Study the drawing (mm; zero at the part's minimum x, y, z) and answer. A direction names the side the tool comes from. Coordinates: 2 decimals unless noted, no trailing zeros. Order: outer loops, then holes, each group sorted by start corner. A loop starts at its lowest first (then second) coordinate and runs counter-clockwise, first axis right, second up.
1. The part is cut by section C-C, the plane y = 2.5. Give the vertices of the cut face in (x, z).
2. The part is cut by section A-A, the plane z = 4.25. Give the vertices of the cut face in (x, y).
3. The part is cut by section D-D, the plane x = 41.5. Give the vertices of the cut face in (y, z), then the cut area to 3 significant figures.
4. The part is cut by section B-B, the plane y = 17.2. Give the vertices of the cut face in (x, z).
5. Find the intervals of material crossed by probe 1 along Z at (x, y) = (2.65, 17.2); probe 2 along X at (y, z) = (9.75, 1.5); probe 3 along Z at (x, y) = (10, 3.5), in increasing order.
6. Determine the mould class of the marked faces 3, 4 and 5 for opening direction X: +X half, -X half, draft (parallel to the pull), parting line (faces both ways), or undercut.
7. A tool of negligible diameter and unlimited length cuts with its end or side. For the marked faces 1 and 2, from which of +Z, -Z, +X, -X, +Y, -Y can it reach the whole face along a straight path? Write none if from no direction.
8. Flat-ended cylindrical pins translate along their axes: pin 1 Ø5 at (x, z) = (42, 4.5) entering from +Y; pin 2 Ø3 at (x, y) = (35, 2.5) entering from -Z; pin 3 Ø4 at (x, z) = (32.5, 5) entering from +Y; pin 4 Ø4.5 at (x, y) = (34.5, 2.5) entering from +Z. Find the tip coordinate at first contact, or state that the pin passes through.
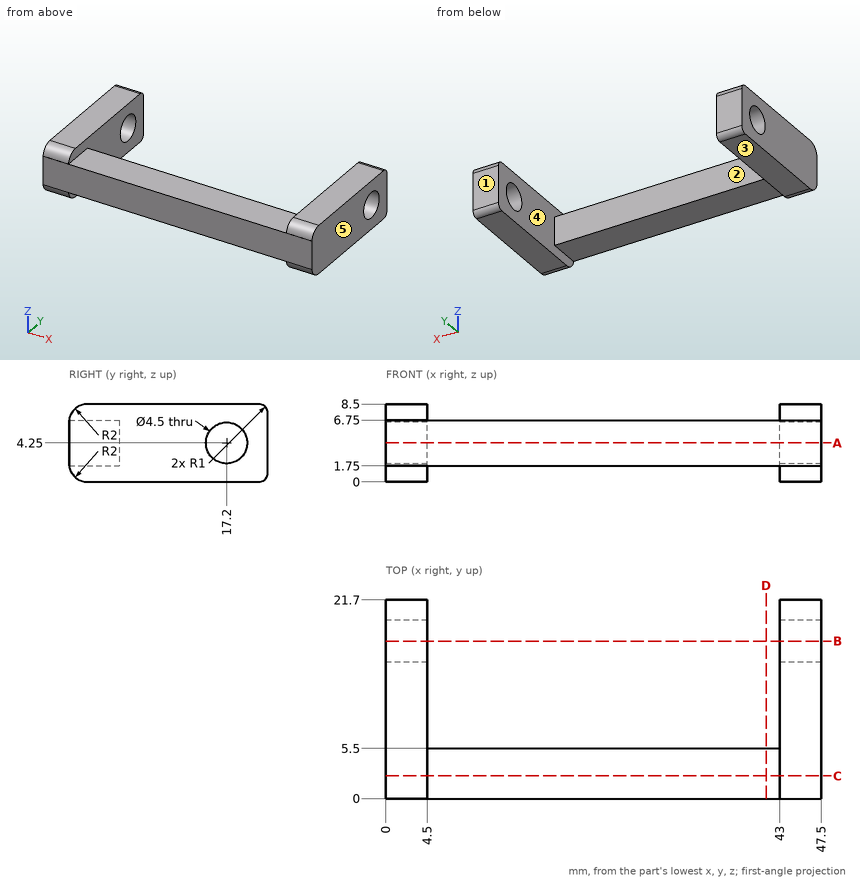
Geometry says:
1. outline: (0, 0) - (4.5, 0) - (4.5, 1.75) - (43, 1.75) - (43, 0) - (47.5, 0) - (47.5, 8.5) - (43, 8.5) - (43, 6.75) - (4.5, 6.75) - (4.5, 8.5) - (0, 8.5) - close
2. outline: (0, 0) - (47.5, 0) - (47.5, 14.95) - (43, 14.95) - (43, 5.5) - (4.5, 5.5) - (4.5, 14.95) - (0, 14.95) - close; (0, 19.45) - (4.5, 19.45) - (4.5, 21.7) - (0, 21.7) - close; (43, 19.45) - (47.5, 19.45) - (47.5, 21.7) - (43, 21.7) - close
3. outline: (0, 1.75) - (5.5, 1.75) - (5.5, 6.75) - (0, 6.75) - close
3. area: 27.5 mm2
4. outline: (0, 0) - (4.5, 0) - (4.5, 2) - (0, 2) - close; (0, 6.5) - (4.5, 6.5) - (4.5, 8.5) - (0, 8.5) - close; (43, 0) - (47.5, 0) - (47.5, 2) - (43, 2) - close; (43, 6.5) - (47.5, 6.5) - (47.5, 8.5) - (43, 8.5) - close
5. probe 1: z = 0 to 2, 6.5 to 8.5
5. probe 2: x = 0 to 4.5, 43 to 47.5
5. probe 3: z = 1.75 to 6.75
6. face 3: draft
6. face 4: undercut
6. face 5: +X half
7. face 1: +Z, -Z, +X, -X, +Y
7. face 2: +Z, -Z, +Y
8. pin 1: stops at y = 21.7
8. pin 2: stops at z = 1.75
8. pin 3: stops at y = 5.5
8. pin 4: stops at z = 6.75
